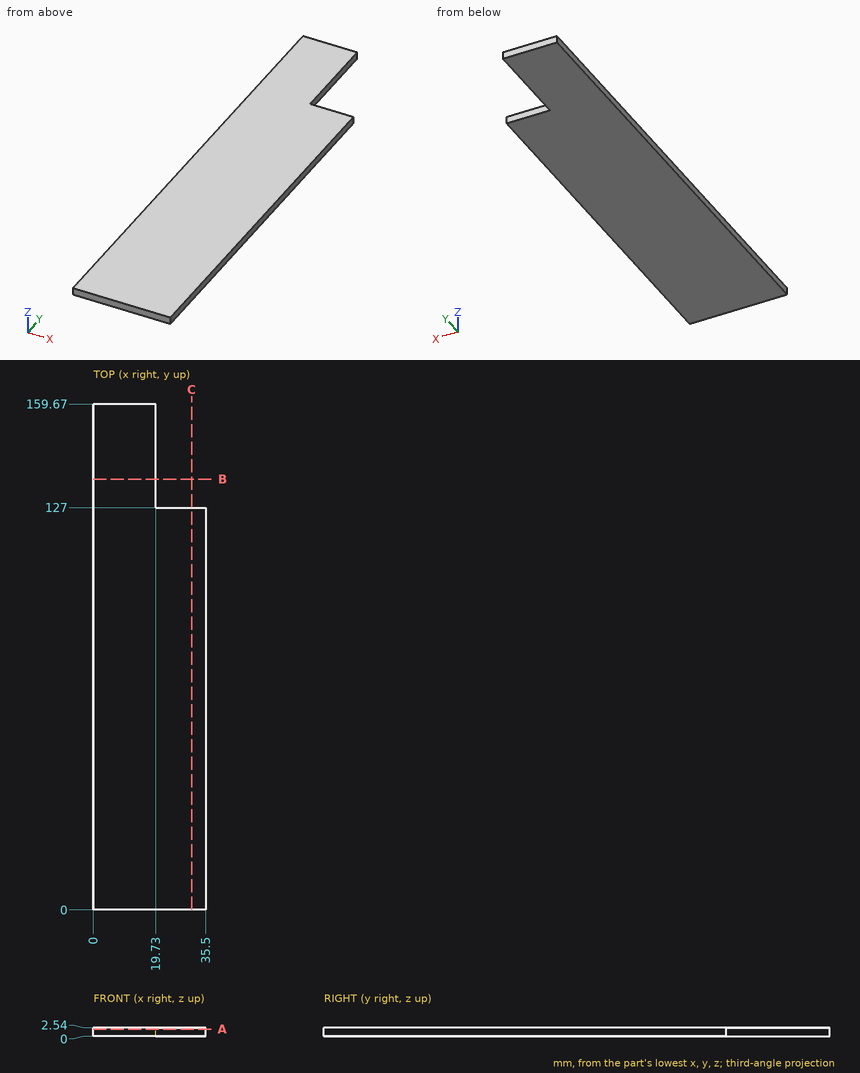
Answer from the drawing. Dimensions are ordinates in mm from the lowest x, y and z of the part. Give positions to 0.01 mm unless a question says otherwise; leave off trailing zeros. Loops run counter-clockwise (first coordinate to the right, second up) from the corner with the lowest first, then second, coordinate; pieces in that order, holes last. Notation, with made-up numbers: (-6, 71.25) - (18, 71.25) arc R26 ccw to (18, 96.25) - close; hole circle Ø11 at (24, -38). An arc over 180 degrees is marked (long way). Write each question's results on one line, items separated by ' | '.
1. Consider probe 1 along Y at (x, z) = (21, 2.3); probe 2 along X at (y, z) = (137, 1). Determine where each line is inside the solid, lowest interval first. Write a range as from..to.
Resolved:
probe 1: y = 0..127 | probe 2: x = 0..19.73
2. Flat-ended cylindrical pins translate along their axes: P1, Ø1.3, axis at x = 26.5, z = 1.5, coming from the +Y side; P2, Ø1.3, axis at y = 149, z = 1, coming from the +X side. Find the tip coordinate at first contact, or state that the pin passes through.
Resolved:
P1: stops at y = 127 | P2: stops at x = 19.73
3. Find section B-B, the plane y = 136. Write down the section's boundary in (x, z), then the cut area to 3 significant figures.
Resolved:
outline: (0, 0) - (19.73, 0) - (19.73, 2.54) - (0, 2.54) - close | area: 50.1 mm^2
4. Find section A-A, the plane z = 2.15. Write down the section's boundary in (x, y).
Resolved:
outline: (0, 0) - (35.5, 0) - (35.5, 127) - (19.73, 127) - (19.73, 159.67) - (0, 159.67) - close
5. Find section C-C, the plane x = 31. Write down the section's boundary in (y, z).
Resolved:
outline: (0, 0) - (127, 0) - (127, 2.54) - (0, 2.54) - close
